```python
from build123d import *

# Parameters (mm, degrees)
F1_DEPTH = 63.5
F0_W     = 25.4
F0_H     = 19.05
F0_H_2   = 4.7498
F0_H_3   = 4.7752
F2_DEPTH = 25.4
F4_DEPTH = 3.175
F5_R     = 12.7


with BuildPart() as f1:
    # F0 (on Front) → F1 (new body, symmetric)
    with BuildSketch(Plane.XZ):
        Polygon((-41.275, -9.525), (41.275, -9.525), (41.275, 9.525), (22.225, 9.525), (-41.275, 9.525), align=None)
    extrude(amount=F1_DEPTH, both=True)

    # F0 (on Front) → F2 (join, symmetric)
    with BuildSketch(Plane.XZ):
        with BuildLine():
            Line((22.225, 9.525), (41.275, 9.525))
            Line((41.275, 9.525), (41.275, 27.0002))
            ThreePointArc((41.275, 27.0002), (45.9246798487, 38.2255201513), (57.15, 42.8752))
            Line((57.15, 42.8752), (60.325, 42.8752))
            Line((60.325, 42.8752), (60.325, 61.9252))
            Line((60.325, 61.9252), (57.15, 61.9252))
            add(Edge.make_bspline(
                [(50.5716827733, 61.3000741611), (52.7396972635, 61.5056461021), (54.9329690535, 61.7131439678), (57.15, 61.9252)],
                knots=[107.178919237, 107.178919237, 107.178919237, 107.178919237, 111.5045361635, 111.5045361635, 111.5045361635, 111.5045361635], degree=3))
            ThreePointArc((50.5716827733, 61.3000741611), (30.2287876003, 49.2488841842), (22.225, 27.0002))
            Line((22.225, 27.0002), (22.225, 9.525))
        make_face()
        with Locations((73.025, 52.4002)):
            Rectangle(F0_W, F0_H)
        with Locations((73.025, 64.3001)):
            Rectangle(F0_W, F0_H_2)
        with Locations((73.025, 40.4876)):
            Rectangle(F0_W, F0_H_3)
    extrude(amount=F2_DEPTH, both=True)

    # F0 (on Front) → F3 (revolve)
    with BuildSketch(Plane.XZ):
        Polygon((85.725, 61.9252), (85.725, 42.8752), (85.725, 38.1), (111.125, 38.1), (111.125, 66.675), (85.725, 66.675), align=None)
    revolve(axis=Axis((85.725, 0, 52.3875), (0, 0, 1)))

    # F0 (on Front) → F4 (join, symmetric)
    with BuildSketch(Plane.XZ):
        with BuildLine():
            add(Edge.make_bspline(
                [(-41.275, 9.525), (-41.358874461, 52.2952599857), (-3.1467703164, 56.2064704424), (50.5716827733, 61.3000741611)],
                knots=[0, 0, 0, 0, 107.178919237, 107.178919237, 107.178919237, 107.178919237], degree=3))
            Line((-41.275, 9.525), (22.225, 9.525))
            Line((22.225, 9.525), (22.225, 27.0002))
            ThreePointArc((22.225, 27.0002), (30.2287876003, 49.2488841842), (50.5716827733, 61.3000741611))
        make_face()
    extrude(amount=F4_DEPTH, both=True)

    # F5
    f5_edges = [f1.edges().sort_by_distance(p)[0] for p in [
        (85.725, 25.4, 52.3875),
        (73.025, 25.4, 66.675),
        (73.025, -25.4, 66.675),
        (111.125, 0, 66.675),
    ]]
    fillet(f5_edges, radius=F5_R)


solid = f1.part
```
Source: CAD feature listing. Evaluate the final solid. Frame: model axes, mm. A direction names the side the tool comes from. Round coordinates to 2 decimals unless told otherwise and drop trailing zeros. Write each loop counter-clockwise with the first axis right and the second up, starting at its lowest first coordinate (ties: lowest second). Pieces come first, ordered by that corner, then holes. Notation, with made-up numbers: M 8,75.5 L 40,75.5 A14 cw 40,98.5 Z; hole C 17.5,7.25 d11. An arc over 180 degrees is marked long. Answer as a JSON object with one key per item and string values. Group by question number.
(1) Reachability of faces 4 (the flat face through (41.275, -1, 4)), 5 (the flat face through (46, -25.4, 42)), 6 (the flat face through (22.225, -14, 18)), 7 (the flat face through (46, 25.4, 42)), 8 (the flat face through (-5, 3.175, 30)) from +Z, -Z, +X, -X, +Y, -Y: full face, straight path, thin tool, end or side. Return the list, or none.
(2) Mould query, pull axis X, two halves, no side actions, for faces 1 (the flat face through (-5, -3.175, 30)), 2 (the cylindrical face through (30.445, 14.132, 49.508)), 3 (the cylindrical face through (45.8, -0.4, 38.1)). Classes: +X half, -X half, draft (parallel to the pull), parting line (faces both ways), or undercut.
(3) Ray query, line 1 (Z direction, x = 34, y = -32.5) (3 decimals); line 2 (X direction, y = 15, z = -2.5) (3 decimals); line 3 (Y direction, x = -4, z = 20.5) (3 decimals). Return the intervals inside material, ascending. Write a range as [from, to].
(4) Section query A-A on z = -4. Output: boundary loops of the cut face in (x, y) (3 decimals).
(5) First-contact query: pin 1 (12 mm diameter, centred on x = 12.5, z = 59, fed in from -Y) (3 decimals); pin 2 (12 mm diameter, centred on x = 45, y = -39, fed in from +Z) (3 decimals); pin 3 (22 mm diameter, centred on x = 68, z = 34, fed in from +Y); pin 4 (2 mm diameter, centred on x = 81, y = 28, fed in from -Z). Flat tips, straight axial feed; report the tip coordinate or a pass-through.
Computed values:
{
 "1": {"face 4": "-Z, +X, +Y, -Y", "face 5": "+Z, +X, -X, -Y", "face 6": "+Z, -X, -Y", "face 7": "+Z, +X, -X, +Y", "face 8": "+Z, -X, +Y"},
 "2": {"face 1": "draft", "face 2": "-X half", "face 3": "undercut"},
 "3": {"line 1": "[-9.525, 9.525]", "line 2": "[-41.275, 41.275]", "line 3": "[-3.175, 3.175]"},
 "4": {"outline": "M -41.275,-63.5 L 41.275,-63.5 L 41.275,63.5 L -41.275,63.5 Z"},
 "5": {"pin 1": "y = -3.175", "pin 2": "z = 9.525", "pin 3": "y = 25.4", "pin 4": "through"}
}
